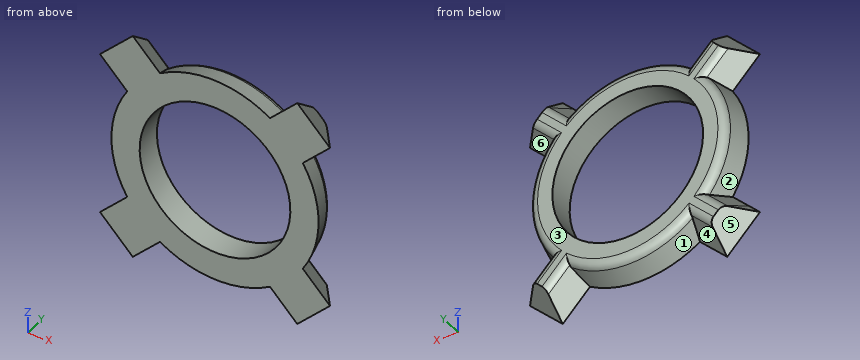
```python
from build123d import *

# Parameters (mm, degrees)
SKETCH2_R           = 12.145554975
BOSS_EXTRUDE1_DEPTH = 3
BOSS_EXTRUDE1_TAPER = 15
BOSS_EXTRUDE2_DEPTH = 3
BOSS_EXTRUDE2_TAPER = 30
FILLET1_R           = 1
CIRPATTERN2_START   = -14.617361382
CIRPATTERN2_DEPTH   = 29.234722764
CIRPATTERN2_START_2 = -0.407249855
CIRPATTERN2_2_DEPTH = 0.81449971
CIRPATTERN2_START_3 = 2.716651032
CIRPATTERN2_3_DEPTH = 13.632761157
CIRPATTERN2_START_4 = -2.716651132
CIRPATTERN2_4_DEPTH = 5.433302164
CIRPATTERN2_START_5 = -11.369329343
CIRPATTERN2_5_DEPTH = 22.738655401
CIRPATTERN2_START_6 = -17
CIRPATTERN2_6_DEPTH = 2.382638618
CIRPATTERN2_START_7 = 14.617361382
CIRPATTERN2_7_DEPTH = 2.382638618
SKETCH4_R           = 8.834020379
CUT_EXTRUDE1_DEPTH  = 20.300641771


with BuildPart() as part:
    # Sketch2 → Boss-Extrude1 (new body)
    with BuildSketch(Plane(origin=(0, 0, 0), x_dir=(1, 0, 0), z_dir=(0, 1, 0))):
        Circle(SKETCH2_R)
    extrude(amount=BOSS_EXTRUDE1_DEPTH, taper=BOSS_EXTRUDE1_TAPER)

    # Sketch3 → Boss-Extrude2 (add)
    with BuildSketch(Plane(origin=(0, 0, 0), x_dir=(1, 0, 0), z_dir=(0, 1, 0))):
        Polygon((-7.65848972, -3.816564986), (-13.481742595, -9.639817861), (-9.639817861, -13.481742595), (-3.816564986, -7.65848972), align=None)
    extrude(amount=BOSS_EXTRUDE2_DEPTH, taper=BOSS_EXTRUDE2_TAPER)

    # Fillet1
    fillet1_edges = [part.edges().sort_by_distance(p)[0] for p in [
        (-8.466560643, 3, 9.858995634),
        (-9.858995634, 3, 8.466560643),
        (-3.880929208, 3, -10.657050022),
    ]]
    fillet(fillet1_edges, radius=FILLET1_R)

    # CirPattern2: read off the stored shape, not the designer's step
    # CirPattern2 outline → CirPattern2 (add)
    with BuildSketch(Plane(origin=(0, 0, 0), x_dir=(0.707106781186545, 0, -0.70710678118655), z_dir=(0.70710678118655, 0, 0.707106781186545)).offset(CIRPATTERN2_START)):
        with BuildLine():
            ThreePointArc((1.273275359, 2.5), (0.907249955, 2.866025404), (0.407249955, 3))
            Line((0.407249955, 3), (-0.407249955, 3))
            ThreePointArc((-0.407249955, 3), (-0.907249955, 2.866025404), (-1.273275359, 2.5))
            Line((-1.273275359, 2.5), (-2.716651032, 0))
            Line((-2.716651032, 0), (2.716651032, 0))
            Line((2.716651032, 0), (1.273275359, 2.5))
        make_face()
    extrude(amount=CIRPATTERN2_DEPTH)

    # CirPattern2 2 outline → CirPattern2 2 (add)
    with BuildSketch(Plane(origin=(0, 0, 0), x_dir=(0.707106781186545, 0, -0.70710678118655), z_dir=(0.70710678118655, 0, 0.707106781186545)).offset(CIRPATTERN2_START_2)):
        with BuildLine():
            Line((16.349412189, 0), (14.617361382, 3))
            Line((14.617361382, 3), (0.407249955, 3))
            ThreePointArc((0.407249955, 3), (0.907249955, 2.866025404), (1.273275359, 2.5))
            Line((1.273275359, 2.5), (2.716651032, 0))
            Line((2.716651032, 0), (16.349412189, 0))
        make_face()
    extrude(amount=CIRPATTERN2_2_DEPTH)

    # CirPattern2 3 outline → CirPattern2 3 (add)
    with BuildSketch(Plane(origin=(0, 0, 0), x_dir=(0.707106781186548, 0, 0.707106781186547), z_dir=(0.707106781186547, 0, -0.707106781186548)).offset(CIRPATTERN2_START_3)):
        with BuildLine():
            Line((2.716651032, 0), (0.407249855, 0))
            Line((0.407249855, 0), (0.407249955, -3))
            ThreePointArc((0.407249955, -3), (0.907249955, -2.866025404), (1.273275359, -2.5))
            Line((1.273275359, -2.5), (2.716651032, 0))
        make_face()
        with BuildLine():
            Line((-0.407249855, 0), (-2.716651032, 0))
            Line((-2.716651032, 0), (-1.273275359, -2.5))
            ThreePointArc((-1.273275359, -2.5), (-0.907249955, -2.866025404), (-0.407249955, -3))
            Line((-0.407249955, -3), (-0.407249855, 0))
        make_face()
    extrude(amount=CIRPATTERN2_3_DEPTH)

    # CirPattern2 4 outline → CirPattern2 4 (add)
    with BuildSketch(Plane(origin=(0, 0, 0), x_dir=(0.707106781186548, 0, 0.707106781186547), z_dir=(0.707106781186547, 0, -0.707106781186548)).offset(CIRPATTERN2_START_4)):
        Polygon((16.349412189, 0), (14.617361382, 0), (14.617361382, -3), align=None)
        Polygon((-14.617361382, 0), (-16.349412189, 0), (-14.617361382, -3), align=None)
    extrude(amount=CIRPATTERN2_4_DEPTH)

    # CirPattern2 5 outline → CirPattern2 5 (cut)
    with BuildSketch(Plane(origin=(0, 0, 0), x_dir=(0.7071067811865451, 0, -0.7071067811865499), z_dir=(0.7071067811865498, 0, 0.7071067811865454)).offset(CIRPATTERN2_START_5)):
        Polygon((14.617361382, 3), (16.349412189, 0), (16.349412189, 3), align=None)
    extrude(amount=CIRPATTERN2_5_DEPTH, mode=Mode.SUBTRACT)

    # CirPattern2 6 outline → CirPattern2 6 (cut)
    with BuildSketch(Plane(origin=(0, 0, 0), x_dir=(0.7071067811865451, 0, -0.7071067811865499), z_dir=(0.7071067811865498, 0, 0.7071067811865454)).offset(CIRPATTERN2_START_6)):
        with BuildLine():
            Line((-0.407249955, 3), (-2.716651132, 3))
            Line((-2.716651132, 3), (-2.716651132, 0))
            Line((-2.716651132, 0), (-1.273275359, 2.5))
            ThreePointArc((-1.273275359, 2.5), (-0.907249955, 2.866025404), (-0.407249955, 3))
        make_face()
        with BuildLine():
            Line((2.716651032, 3), (0.407249955, 3))
            ThreePointArc((0.407249955, 3), (0.907249955, 2.866025404), (1.273275359, 2.5))
            Line((1.273275359, 2.5), (2.716651032, 0))
            Line((2.716651032, 0), (2.716651032, 3))
        make_face()
    extrude(amount=CIRPATTERN2_6_DEPTH, mode=Mode.SUBTRACT)

    # CirPattern2 7 outline → CirPattern2 7 (cut)
    with BuildSketch(Plane(origin=(0, 0, 0), x_dir=(0.7071067811865451, 0, -0.7071067811865499), z_dir=(0.7071067811865498, 0, 0.7071067811865454)).offset(CIRPATTERN2_START_7)):
        with BuildLine():
            Line((-0.407249955, 3), (-2.716651132, 3))
            Line((-2.716651132, 3), (-2.716651132, 0))
            Line((-2.716651132, 0), (-1.273275359, 2.5))
            ThreePointArc((-1.273275359, 2.5), (-0.907249955, 2.866025404), (-0.407249955, 3))
        make_face()
        with BuildLine():
            Line((2.716651032, 3), (0.407249955, 3))
            ThreePointArc((0.407249955, 3), (0.907249955, 2.866025404), (1.273275359, 2.5))
            Line((1.273275359, 2.5), (2.716651032, 0))
            Line((2.716651032, 0), (2.716651032, 3))
        make_face()
    extrude(amount=CIRPATTERN2_7_DEPTH, mode=Mode.SUBTRACT)

    # Sketch4 → Cut-Extrude1 (cut, through all)
    with BuildSketch(Plane(origin=(0, 3, 0), x_dir=(1, 0, 0), z_dir=(0, 1, 0))):
        with Locations(Location((0, 0, 0), (0, 0, 270))):
            Circle(SKETCH4_R)
    extrude(amount=-CUT_EXTRUDE1_DEPTH, mode=Mode.SUBTRACT)


solid = part.part
```
Geometry: final body of the model. Coordinates: model frame, mm. Face numbers are marked on the shaded views. A direction names the side the tool comes from. Round coordinates to 2 decimals unless told otherwise and drop trailing zeros. Order: outer loops, then holes, each group sorted by start corner. A loop starts at its lowest first (then second) coordinate and runs counter-clockwise, first axis right, second up. Notation, with made-up numbers: (12, -33) -> (44, -33) arc R31 cw to (44, 2) -> close; hole circle Ø11 at (23, -33). An arc over 180 degrees is marked (long way). Use one line per item in the form item = value.
(1) Ray query, probe 1 along Z at (x, y) = (-4, 2.1); probe 2 along X at (y, z) = (1.3, 0); probe 3 along Z at (x, y) = (10.75, 1.6). Return the intervals inside material, ascending. Write a range as [from, to].
Results list:
probe_1 = [-10.87, -7.88], [7.88, 10.87]
probe_2 = [-11.8, -8.83], [8.83, 11.8]
probe_3 = [-11.07, -8.21], [-4.66, 4.66], [8.21, 11.07]
(2) Draft query along Z for the marked faces 1, 2 and 3. Return one class per face: pulls with the +Z half, pulls with the -Z half, needs draft (parallel to the pull), parting line crosses it, or undercut.
Results list:
face_1 = pulls with the -Z half
face_2 = undercut
face_3 = needs draft
(3) Section A-A on z = 0. Return loops of the section in (x, y), and give its area (3 significant figures).
Results list:
outline = (-12.15, 0) -> (-8.83, 0) -> (-8.83, 3) -> (-10.57, 3) arc R1 ccw to (-11.54, 2.26) -> close; (8.83, 0) -> (12.15, 0) -> (11.54, 2.26) arc R1 ccw to (10.57, 3) -> (8.83, 3) -> close
area = 17.2 mm^2
(4) Access query for the marked faces 4, 5 and 6. Directions: +Z, -Z, +X, -X, +Y, -Y. A direction counts if a zero-diameter tool reaches every point of the face in a straight line with its end or side. Return the directions, or none.
Results list:
face_4 = -Z, +Y
face_5 = -Z, -X, +Y
face_6 = +X, +Y
(5) First-contact query: pin 1 Ø1 at (x, y) = (-1.5, 2) entering from -Z. Flat tip, straight axial feed; report the tip coordinate or a pass-through.
Results list:
pin_1 = -11.66
(6) Section B-B on x = 0. Return loops of the section in (y, z).
Results list:
outline = (0, -12.15) -> (2.26, -11.54) arc R1 ccw to (3, -10.57) -> (3, -8.83) -> (0, -8.83) -> close; (0, 8.83) -> (3, 8.83) -> (3, 10.57) arc R1 ccw to (2.26, 11.54) -> (0, 12.15) -> close
